```python
from build123d import *

# Parameters (mm, degrees)
BASE_FLANGE1_DEPTH   = 997
CUT_EXTRUDE1_DEPTH   = 10
SKETCH7_R            = 225
CUT_EXTRUDE2_DEPTH   = 10
SKETCH8_R            = 4
CUT_EXTRUDE3_DEPTH   = 10
CUT_EXTRUDE4_DEPTH   = 10
LPATTERN1_COUNT      = 3
LPATTERN1_PITCH      = 375
LPATTERN1_COUNT_DIR2 = 2
LPATTERN1_PITCH_DIR2 = 564.02
CHAMFER1_SIZE        = 4


# Sheet-metal steps are written as plain solids
with BuildPart() as part:
    # Sketch1 → Base-Flange1 (new body)
    with BuildSketch(Plane(origin=(0, 0, 0), x_dir=(1, 0, 0), z_dir=(0, 1, 0))):
        with BuildLine():
            Line((116.152236891, -603), (297.071067812, -422.08116908))
            ThreePointArc((297.071067812, -422.08116908), (299.238795325, -418.836935591), (300, -415.010101268))
            Line((300, -415.010101268), (300, 211.010101268))
            ThreePointArc((300, 211.010101268), (299.238795325, 214.836935591), (297.071067812, 218.08116908))
            Line((297.071067812, 218.08116908), (119.08116908, 396.071067812))
            ThreePointArc((119.08116908, 396.071067812), (115.836935591, 398.238795325), (112.010101268, 399))
            Line((112.010101268, 399), (-516, 399))
            Line((-516, 399), (-516, 395))
            Line((-516, 395), (112.010101268, 395))
            ThreePointArc((112.010101268, 395), (114.306201862, 394.543277195), (116.252741955, 393.242640687))
            Line((116.252741955, 393.242640687), (294.242640687, 215.252741955))
            ThreePointArc((294.242640687, 215.252741955), (295.543277195, 213.306201862), (296, 211.010101268))
            Line((296, 211.010101268), (296, -415.010101268))
            ThreePointArc((296, -415.010101268), (295.543277195, -417.306201862), (294.242640687, -419.252741955))
            Line((294.242640687, -419.252741955), (113.323809767, -600.171572875))
            Line((113.323809767, -600.171572875), (116.152236891, -603))
        make_face()
    extrude(amount=BASE_FLANGE1_DEPTH)

    # Sketch6 → Cut-Extrude1 (cut)
    with BuildSketch(Plane(origin=(257.576118446, 0, -257.576118446), x_dir=(-0.7071067811865485, 0, -0.7071067811865466), z_dir=(0.7071067811865466, 0, -0.7071067811865485))):
        with BuildLine():
            Line((-30.138564286, 134), (-30.138564286, 234))
            ThreePointArc((-30.138564286, 234), (69.861435714, 334), (169.861435714, 234))
            Line((169.861435714, 234), (169.861435714, 134))
            ThreePointArc((169.861435714, 134), (69.861435714, 34), (-30.138564286, 134))
        make_face()
    extrude(amount=-CUT_EXTRUDE1_DEPTH, mode=Mode.SUBTRACT)

    # Sketch7 → Cut-Extrude2 (cut)
    with BuildSketch(Plane(origin=(0, 0, -399), x_dir=(-1, 0, 0), z_dir=(0, 0, -1))):
        with Locations((204, 255)):
            Circle(SKETCH7_R)
    extrude(amount=-CUT_EXTRUDE2_DEPTH, mode=Mode.SUBTRACT)

    # Sketch8 → Cut-Extrude3 (cut)
    with BuildSketch(Plane(origin=(300, 0, 0), x_dir=(0, 0, -1), z_dir=(1, 0, 0))):
        with Locations((180.010101268, 873.5)):
            Circle(SKETCH8_R)
    cut_extrude3 = extrude(amount=-CUT_EXTRUDE3_DEPTH, mode=Mode.SUBTRACT)

    # Sketch9 → Cut-Extrude4 (cut)
    with BuildSketch(Plane(origin=(359.576118446, 0, 359.576118446), x_dir=(0.7071067811865415, 0, -0.7071067811865536), z_dir=(0.7071067811865536, 0, 0.7071067811865415))):
        with BuildLine():
            Line((-314.395490323, 134), (-314.395490323, 234))
            ThreePointArc((-314.395490323, 234), (-214.395490323, 334), (-114.395490323, 234))
            Line((-114.395490323, 234), (-114.395490323, 134))
            ThreePointArc((-114.395490323, 134), (-214.395490323, 34), (-314.395490323, 134))
        make_face()
    extrude(amount=-CUT_EXTRUDE4_DEPTH, mode=Mode.SUBTRACT)

    # LPattern1: Cut-Extrude3 3 × 2
    with Locations(*[(0, -i * LPATTERN1_PITCH, j * LPATTERN1_PITCH_DIR2) for i in range(LPATTERN1_COUNT) for j in range(LPATTERN1_COUNT_DIR2) if (i, j) != (0, 0)]):
        add(cut_extrude3, mode=Mode.SUBTRACT)

    # Chamfer1
    chamfer1_edges = [part.edges().sort_by_distance(p)[0] for p in [
        (-516, 498.5, -399),
        (116.152236891, 498.5, 603),
    ]]
    chamfer(chamfer1_edges, length=CHAMFER1_SIZE - 0.0001)  # a hair under: the kernel refuses the full size


solid = part.part
```
The listing builds one solid part. Answer for the finished solid, in the listing's coordinates (mm). A direction names the side the tool comes from. Round coordinates to 2 decimals unless told otherwise and drop trailing zeros. Loops run counter-clockwise (first coordinate to the right, second up) from the corner with the lowest first, then second, coordinate; pieces in that order, holes last. Notation, with made-up numbers: (67.5, -25.75) - (82.5, -25.75) arc R6 cw to (82.5, -21.75) - close; hole circle Ø1 at (86, 84.5). An arc over 180 degrees is marked (long way). Use one line per item in the form item = value. Start each with the question number.
1. Consider line 1 (Z direction, x = 297, y = 123); line 2 (Y direction, x = -204, z = -397); line 3 (Z direction, x = 299, y = 873.5). Determine where each line is inside the solid, lowest interval first. Write a range as [from, to].
2. The part is cut by section A-A on x = -204. Determine the outline of the cut face in (y, z), then the cut area to 3 significant figures.
3. For a pull along Y with two mould halves and no side action, classify faces 6 (the face through (204.002, 602.299, -305.494)), 7 (the face through (-174.709, 478.085, -397.028)) as pulls with the +Y half, pulls with the -Y half, needs draft (parallel to the pull), parting line crosses it, or undercut.
4. The part is cut by section D-D on z = 48.5. Determine the outline of the cut face in (x, y), then the cut area to 3 significant figures.
5. Given pin 1 Ø12 at (x, y) = (-138.5, 689.5) entering from +Z; pin 2 Ø9 at (y, z) = (498.5, -180.01) entering from -X; pin 3 Ø5 at (y, z) = (873.5, -180.01) entering from +X; pin 4 Ø12 at (x, y) = (149, 503) entering from -Z, each flat-ended and moving along its own axis, determine where each tip first touches the part or whether it passes through.
6. The part is cut by section B-B on y = 91.5. Give the number of separate pieces and of enclosed holes in the cut face, then the cut area to 3 significant figures.
7. A tool of negligible diameter and unlimited length cuts with its end or side. For faces 1 (the face through (296, 492, 98)), 2 (the face through (-196, 602, -399)), 3 (the face through (-206, 602, -395)), 4 (the face through (205.026, 333.976, 511.337)), 5 (the face through (300, 492, 106)), from which of +Z, -Z, +X, -X, +Y, -Y can it reach the whole face along a straight path? Write none if from no direction.
Geometry check:
q1.line_1 = [-218.15, -183.98], [-176.04, 380.04], [387.98, 422.15]
q1.line_2 = [0, 30], [480, 997]
q1.line_3 = [-215.37, -184.01], [-176.01, 380.01], [388.01, 419.37]
q2.outline = (0, -399) - (30, -399) - (30, -395) - (0, -395) - close; (480, -399) - (997, -399) - (997, -395) - (480, -395) - close
q2.area = 2,190 mm^2
q3.face_6 = needs draft
q3.face_7 = undercut
q4.outline = (296, 0) - (300, 0) - (300, 997) - (296, 997) - close
q4.area = 3,990 mm^2
q5.pin_1 = -395
q5.pin_2 = 296
q5.pin_3 = through
q5.pin_4 = -372.15
q6.separate_pieces = 4
q6.enclosed_holes = 0
q6.area = 4,420 mm^2
q7.face_1 = -X, +Y, -Y
q7.face_2 = -Z, +X, -X, +Y, -Y
q7.face_3 = +Z, -X, +Y, -Y
q7.face_4 = none
q7.face_5 = +Z, -Z, +X, +Y, -Y
